Here's how the part is built. I have some questions about the finished solid (model axes, mm). Face numbers are marked on the shaded views. A direction names the side the tool comes from. Coordinates: 2 decimals unless noted, no trailing zeros. Write each loop counter-clockwise with the first axis right and the second up, starting at its lowest first coordinate (ties: lowest second). Pieces come first, ordered by that corner, then holes. Notation, with made-up numbers: (22.5, 58.5) -> (53.5, 58.5) arc R19 ccw to (53.5, 93.5) -> close; hole circle Ø10 at (48, 69.5). An arc over 180 degrees is marked (long way). Use a Markdown table: item, result. Add a question column.
Item 1: On a 3-axis mill with a long thin cutter (end or side, diameter ignored), from which of +Z, -Z, +X, -X, +Y, -Y can I reach the whole of each face in a straight line? I mean the marked faces 1 and 2. Say none if no direction works.
Item 2: Imagine slicing it at C-C, the plane y = 2.25. Write out the boundary of the cut face in (x, z), and give its area (3 significant figures).
Item 3: Imagine slicing it at B-B, the plane x = 1. Write out the boundary of the cut face in (y, z), and give its area (3 significant figures).
Item 4: Imagine slicing it at D-D, the plane x = -2.5. Write out the boundary of the cut face in (y, z).
Item 5: Imagine slicing it at A-A, the plane y = 0.25. Write out the boundary of the cut face in (x, z), and give its area (3 significant figures).
Item 6: If we mould it in two halves opening along X, with no side actions, what happens to the marked faces 3, 4 and 5? For each: pulls with the +X half, pulls with the -X half, needs draft (parallel to the pull), parting line crosses it, or undercut.
Item 7: If I drill on line 1 along Z through (x, y) = (-1.25, -3.5); line 2 along Y through (x, z) = (-0.25, 9.5); line 3 along X through (y, z) = (-1.25, 10.5), over which ranges is the centre line in solid material (lowest first)? Write a range as from..to.
Item 8: Will these pins go through, and if not, where does the flat tip stop? pin 1 Ø4.5 at (x, y) = (-1, -1) entering from -Z; pin 2 Ø1 at (y, z) = (1.5, 13.5) entering from +X; pin 3 Ø3 at (x, z) = (-3, 15.5) entering from -Y.
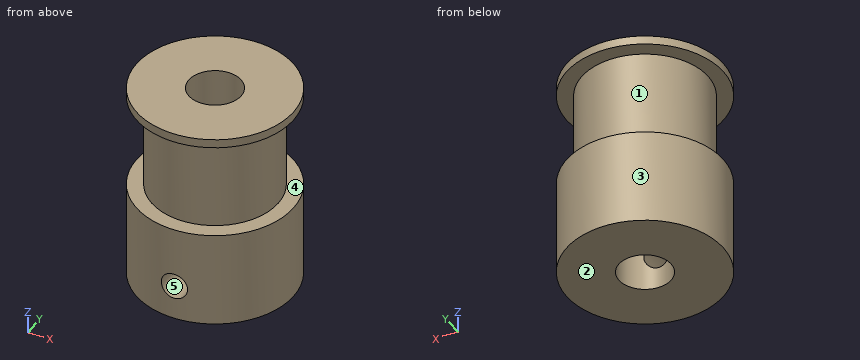
```python
from build123d import *

# Parameters (mm, degrees)
SKETCH1_R           = 9
SKETCH1_R_2         = 3
BOSS_EXTRUDE1_DEPTH = 11.05
SKETCH2_R           = 7.25
SKETCH2_R_2         = 3
BOSS_EXTRUDE2_DEPTH = 11
SKETCH3_R           = 9
SKETCH3_R_2         = 3
BOSS_EXTRUDE3_DEPTH = 1
SKETCH4_R           = 1.5
CUT_EXTRUDE1_DEPTH  = 27.330638048
ECHELLE1_SCALE      = 2
ECHELLE2_SCALE      = 0.25


with BuildPart() as part:
    # Sketch1 → Boss-Extrude1 (new body)
    with BuildSketch(Plane.XY):
        Circle(SKETCH1_R)
        Circle(SKETCH1_R_2, mode=Mode.SUBTRACT)
    extrude(amount=BOSS_EXTRUDE1_DEPTH)

    # Sketch2 → Boss-Extrude2 (add)
    with BuildSketch(Plane.XY.offset(11.05)):
        Circle(SKETCH2_R)
        Circle(SKETCH2_R_2, mode=Mode.SUBTRACT)
    extrude(amount=BOSS_EXTRUDE2_DEPTH)

    # Sketch3 → Boss-Extrude3 (add)
    with BuildSketch(Plane.XY.offset(22.05)):
        Circle(SKETCH3_R)
        Circle(SKETCH3_R_2, mode=Mode.SUBTRACT)
    extrude(amount=BOSS_EXTRUDE3_DEPTH)

    # Sketch4 → Cut-Extrude1 (cut, through all)
    with BuildSketch(Plane(origin=(0, 0, 0), x_dir=(1, 0, 0), z_dir=(0, 1, 0))):
        with Locations(Location((0, -4, 0), (0, 0, 270))):
            Circle(SKETCH4_R)
    extrude(amount=-CUT_EXTRUDE1_DEPTH, mode=Mode.SUBTRACT)


with BuildPart() as part_1:
    # Echelle1: scaled about (3.613e-06, 0.060757241, 10.422968187)
    add(part.part.scale(ECHELLE1_SCALE).moved(Location((-3.613e-06, -0.060757241, -10.422968187))))


with BuildPart() as part_2:
    # Echelle2: scaled about (3.614e-06, 0.060757242, 10.422968188)
    add(part_1.part.scale(ECHELLE2_SCALE).moved(Location((2.711e-06, 0.045567932, 7.817226141))))


solid = part_2.part
```
Ans:
| question | item | result |
|---|---|---|
| 1 | face 1 | none |
| 1 | face 2 | -Z, +X, -X, +Y, -Y |
| 2 | outline | (-3.91, 5.21) -> (3.91, 5.21) -> (3.91, 10.74) -> (2.87, 10.74) -> (2.87, 16.24) -> (3.91, 16.24) -> (3.91, 16.74) -> (-3.91, 16.74) -> (-3.91, 16.24) -> (-2.87, 16.24) -> (-2.87, 10.74) -> (-3.91, 10.74) -> close |
| 2 | area | 78.7 mm^2 |
| 3 | outline | (-4.36, 5.21) -> (-1.09, 5.21) -> (-1.09, 16.74) -> (-4.36, 16.74) -> (-4.36, 16.24) -> (-3.45, 16.24) -> (-3.45, 10.74) -> (-4.36, 10.74) -> close; (1.15, 5.21) -> (4.42, 5.21) -> (4.42, 10.74) -> (3.51, 10.74) -> (3.51, 16.24) -> (4.42, 16.24) -> (4.42, 16.74) -> (1.15, 16.74) -> close |
| 3 | area | 65.4 mm^2 |
| 4 | outline | (-3.71, 5.21) -> (3.77, 5.21) -> (3.77, 10.74) -> (2.66, 10.74) -> (2.66, 16.24) -> (3.77, 16.24) -> (3.77, 16.74) -> (-3.71, 16.74) -> (-3.71, 16.24) -> (-2.59, 16.24) -> (-2.59, 10.74) -> (-3.71, 10.74) -> close |
| 5 | outline | (-4.49, 5.21) -> (-1.48, 5.21) -> (-1.48, 16.74) -> (-4.49, 16.74) -> (-4.49, 16.24) -> (-3.62, 16.24) -> (-3.62, 10.74) -> (-4.49, 10.74) -> close; (1.48, 5.21) -> (4.49, 5.21) -> (4.49, 10.74) -> (3.62, 10.74) -> (3.62, 16.24) -> (4.49, 16.24) -> (4.49, 16.74) -> (1.48, 16.74) -> close |
| 5 | area | 59.8 mm^2 |
| 6 | face 3 | parting line crosses it |
| 6 | face 4 | needs draft |
| 6 | face 5 | undercut |
| 7 | line 1 | z = 5.21..10.74, 16.24..16.74 |
| 7 | line 2 | y = -4.46..-1.45, 1.51..4.52 |
| 7 | line 3 | x = -4.31..-0.78, 0.78..4.31 |
| 8 | pin 1 | stops at z = 5.21 |
| 8 | pin 2 | stops at x = 3.49 |
| 8 | pin 3 | stops at y = -4.14 |
